The listing builds one solid part. Answer for the finished solid, in the listing's coordinates (mm). Give positions to 0.01 mm unless a question says otherwise; leave off trailing zeros. Write each loop counter-clockwise with the first axis right and the second up, starting at its lowest first coordinate (ties: lowest second). Pieces come first, ordered by that corner, then holes. Notation, with made-up numbers: (-16.75, 79.25) - (-0.75, 79.25) arc R18 cw to (-0.75, 85.25) - close; hole circle Ø11 at (-3.5, 23). An arc over 180 degrees is marked (long way). Use a Markdown table: item, result. Add a question column.
from build123d import *

# Parameters (mm, degrees)
SKETCH_1_W      = 150
SKETCH_1_H      = 100
SKETCH_1_R      = 39
SKETCH_1_R_2    = 1.5
SKETCH_1_R_3    = 1.65
EXTRUDE_1_DEPTH = 3


with BuildPart() as part:
    # 草图1 → 凸台-拉伸1 (new body)
    with BuildSketch(Plane.XY):
        Rectangle(SKETCH_1_W, SKETCH_1_H)
        Circle(SKETCH_1_R, mode=Mode.SUBTRACT)
        with Locations((42.5, 0)):
            Circle(SKETCH_1_R_2, mode=Mode.SUBTRACT)
        with Locations((30.0520382, -30.0520382)):
            Circle(SKETCH_1_R_2, mode=Mode.SUBTRACT)
        with Locations((0, -42.5)):
            Circle(SKETCH_1_R_2, mode=Mode.SUBTRACT)
        with Locations((-30.0520382, -30.0520382)):
            Circle(SKETCH_1_R_2, mode=Mode.SUBTRACT)
        with Locations((-42.5, 0)):
            Circle(SKETCH_1_R_2, mode=Mode.SUBTRACT)
        with Locations((-30.0520382, 30.0520382)):
            Circle(SKETCH_1_R_2, mode=Mode.SUBTRACT)
        with Locations((0, 42.5)):
            Circle(SKETCH_1_R_2, mode=Mode.SUBTRACT)
        with Locations((30.0520382, 30.0520382)):
            Circle(SKETCH_1_R_2, mode=Mode.SUBTRACT)
        with Locations((-65, 30)):
            Circle(SKETCH_1_R_3, mode=Mode.SUBTRACT)
        with Locations((-65, 10)):
            Circle(SKETCH_1_R_3, mode=Mode.SUBTRACT)
        with Locations((-65, -10)):
            Circle(SKETCH_1_R_3, mode=Mode.SUBTRACT)
        with Locations((-65, -30)):
            Circle(SKETCH_1_R_3, mode=Mode.SUBTRACT)
        with Locations(Location((65, -30, 0), (0, 0, 180))):
            Circle(SKETCH_1_R_3, mode=Mode.SUBTRACT)
        with Locations(Location((65, -10, 0), (0, 0, 180))):
            Circle(SKETCH_1_R_3, mode=Mode.SUBTRACT)
        with Locations(Location((65, 10, 0), (0, 0, 180))):
            Circle(SKETCH_1_R_3, mode=Mode.SUBTRACT)
        with Locations(Location((65, 30, 0), (0, 0, 180))):
            Circle(SKETCH_1_R_3, mode=Mode.SUBTRACT)
    extrude(amount=EXTRUDE_1_DEPTH)


solid = part.part
1. For a pull along Y with two mould halves and no side action, classify faces 1 (the flat face through (-1, 50, 1)), 2 (the cylindrical face through (-66.216, 31.115, 1.479)), 3 (the flat face through (-34, 23, 0)), 4 (the cylindrical face through (41, 0, 1)) as released by +Y, released by -Y, zero draft, split by the parting line, or undercut.
2. The part is cut by section B-B (x = -65). Give the vertices of the cut face in (y, z), and give its area (3 significant figures).
3. Consider L1, parallel to Y at x = 0, z = 1.7; L2, parallel to Y at x = -42.5, z = 1.3; L3, parallel to Y at x = 65, z = 0.75. Determine where each line is inside the solid, lowest interval first. Write a range as [from, to].
4. The part is cut by section C-C (y = -36). Give the vertices of the cut face in (x, z).
5. The part is cut by section D-D (x = 42.5). Give the vertices of the cut face in (y, z).
6. The part is cut by section A-A (y = 0). Give the vertices of the cut face in (x, z), and give its area (3 significant figures).
Check values:
| question | item | result |
|---|---|---|
| 1 | face 1 | released by +Y |
| 1 | face 2 | undercut |
| 1 | face 3 | zero draft |
| 1 | face 4 | undercut |
| 2 | outline | (-50, 0) - (-31.65, 0) - (-31.65, 3) - (-50, 3) - close; (-28.35, 0) - (-11.65, 0) - (-11.65, 3) - (-28.35, 3) - close; (-8.35, 0) - (8.35, 0) - (8.35, 3) - (-8.35, 3) - close; (11.65, 0) - (28.35, 0) - (28.35, 3) - (11.65, 3) - close; (31.65, 0) - (50, 0) - (50, 3) - (31.65, 3) - close |
| 2 | area | 260 mm2 |
| 3 | L1 | y = [-50, -44], [-41, -39], [39, 41], [44, 50] |
| 3 | L2 | y = [-50, -1.5], [1.5, 50] |
| 3 | L3 | y = [-50, -31.65], [-28.35, -11.65], [-8.35, 8.35], [11.65, 28.35], [31.65, 50] |
| 4 | outline | (-75, 0) - (-15, 0) - (-15, 3) - (-75, 3) - close; (15, 0) - (75, 0) - (75, 3) - (15, 3) - close |
| 5 | outline | (-50, 0) - (-1.5, 0) - (-1.5, 3) - (-50, 3) - close; (1.5, 0) - (50, 0) - (50, 3) - (1.5, 3) - close |
| 6 | outline | (-75, 0) - (-44, 0) - (-44, 3) - (-75, 3) - close; (-41, 0) - (-39, 0) - (-39, 3) - (-41, 3) - close; (39, 0) - (41, 0) - (41, 3) - (39, 3) - close; (44, 0) - (75, 0) - (75, 3) - (44, 3) - close |
| 6 | area | 198 mm2 |
